```python
from build123d import *

# Parameters (mm, degrees)
CUT_EXTRUDE1_REACH = 53.976
SKETCH2_R          = 3
SKETCH2_R_2        = 2.6


with BuildPart() as part:
    # Sketch1 → Revolve1 (revolve)
    with BuildSketch(Plane.XY, mode=Mode.PRIVATE) as revolve1_sk:
        Polygon((0, -15.5), (29.5, -15.5), (29.5, -9.5), (15, -9.5), (15, 15.5), (0, 15.5), align=None)
    revolve(revolve1_sk.sketch.rotate(Axis((0, 0, 0), (0, -1, 0)), 180), axis=Axis((0, 0, 0), (0, -1, 0)))

    # Sketch2 → Cut-Extrude1 (cut, up to next)
    with BuildSketch(Plane(origin=(0, 15.5, 0), x_dir=(1, 0, 0), z_dir=(0, 1, 0)), mode=Mode.PRIVATE) as cut_extrude1_sk1:
        with Locations(Location((0, 0, 0), (0, 0, 180))):
            Circle(SKETCH2_R)
    cut_extrude1_tool1 = extrude(cut_extrude1_sk1.sketch, amount=-CUT_EXTRUDE1_REACH, mode=Mode.PRIVATE) & part.part
    # Sketch2 → Cut-Extrude1 (cut, up to next)
    with BuildSketch(Plane(origin=(0, 15.5, 0), x_dir=(1, 0, 0), z_dir=(0, 1, 0)), mode=Mode.PRIVATE) as cut_extrude1_sk2:
        with Locations(Location((0, 23.75, 0), (0, 0, 180))):
            Circle(SKETCH2_R_2)
    cut_extrude1_tool2 = extrude(cut_extrude1_sk2.sketch, amount=-CUT_EXTRUDE1_REACH, mode=Mode.PRIVATE) & part.part
    # Sketch2 → Cut-Extrude1 (cut, up to next)
    with BuildSketch(Plane(origin=(0, 15.5, 0), x_dir=(1, 0, 0), z_dir=(0, 1, 0)), mode=Mode.PRIVATE) as cut_extrude1_sk3:
        with Locations(Location((20.56810334, 11.875, 0), (0, 0, 180))):
            Circle(SKETCH2_R_2)
    cut_extrude1_tool3 = extrude(cut_extrude1_sk3.sketch, amount=-CUT_EXTRUDE1_REACH, mode=Mode.PRIVATE) & part.part
    # Sketch2 → Cut-Extrude1 (cut, up to next)
    with BuildSketch(Plane(origin=(0, 15.5, 0), x_dir=(1, 0, 0), z_dir=(0, 1, 0)), mode=Mode.PRIVATE) as cut_extrude1_sk4:
        with Locations(Location((20.56810334, -11.875, 0), (0, 0, 180))):
            Circle(SKETCH2_R_2)
    cut_extrude1_tool4 = extrude(cut_extrude1_sk4.sketch, amount=-CUT_EXTRUDE1_REACH, mode=Mode.PRIVATE) & part.part
    # Sketch2 → Cut-Extrude1 (cut, up to next)
    with BuildSketch(Plane(origin=(0, 15.5, 0), x_dir=(1, 0, 0), z_dir=(0, 1, 0)), mode=Mode.PRIVATE) as cut_extrude1_sk5:
        with Locations(Location((0, -23.75, 0), (0, 0, 180))):
            Circle(SKETCH2_R_2)
    cut_extrude1_tool5 = extrude(cut_extrude1_sk5.sketch, amount=-CUT_EXTRUDE1_REACH, mode=Mode.PRIVATE) & part.part
    # Sketch2 → Cut-Extrude1 (cut, up to next)
    with BuildSketch(Plane(origin=(0, 15.5, 0), x_dir=(1, 0, 0), z_dir=(0, 1, 0)), mode=Mode.PRIVATE) as cut_extrude1_sk6:
        with Locations(Location((-20.56810334, -11.875, 0), (0, 0, 180))):
            Circle(SKETCH2_R_2)
    cut_extrude1_tool6 = extrude(cut_extrude1_sk6.sketch, amount=-CUT_EXTRUDE1_REACH, mode=Mode.PRIVATE) & part.part
    # Sketch2 → Cut-Extrude1 (cut, up to next)
    with BuildSketch(Plane(origin=(0, 15.5, 0), x_dir=(1, 0, 0), z_dir=(0, 1, 0)), mode=Mode.PRIVATE) as cut_extrude1_sk7:
        with Locations(Location((-20.56810334, 11.875, 0), (0, 0, 180))):
            Circle(SKETCH2_R_2)
    cut_extrude1_tool7 = extrude(cut_extrude1_sk7.sketch, amount=-CUT_EXTRUDE1_REACH, mode=Mode.PRIVATE) & part.part
    add(cut_extrude1_tool1.solids().sort_by_distance((0, 15.5, 0))[0], mode=Mode.SUBTRACT)
    add(cut_extrude1_tool2.solids().sort_by_distance((0, 15.5, -23.75))[0], mode=Mode.SUBTRACT)
    add(cut_extrude1_tool3.solids().sort_by_distance((20.568103, 15.5, -11.875))[0], mode=Mode.SUBTRACT)
    add(cut_extrude1_tool4.solids().sort_by_distance((20.568103, 15.5, 11.875))[0], mode=Mode.SUBTRACT)
    add(cut_extrude1_tool5.solids().sort_by_distance((0, 15.5, 23.75))[0], mode=Mode.SUBTRACT)
    add(cut_extrude1_tool6.solids().sort_by_distance((-20.568103, 15.5, 11.875))[0], mode=Mode.SUBTRACT)
    add(cut_extrude1_tool7.solids().sort_by_distance((-20.568103, 15.5, -11.875))[0], mode=Mode.SUBTRACT)


solid = part.part
```
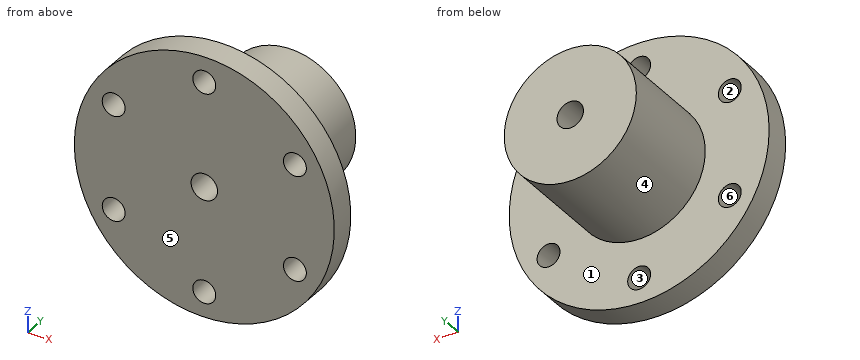
Could you check a few things on this model? Use its own coordinates, in mm. Face numbers are marked on the shaded views. A direction names the side the tool comes from. Round coordinates to 2 decimals unless told otherwise and drop trailing zeros. Order: outer loops, then holes, each group sorted by start corner. A loop starts at its lowest first (then second) coordinate and runs counter-clockwise, first axis right, second up. Notation, with made-up numbers: M 30,-12.75 L 68,-12.75 A11 ccw 68,1.25 Z; hole C 0.5,37.5 d11. An arc over 180 degrees is marked long. One line per question, with ' | ' between items. Start each with the question number.
(1) Suppose I cut it at B-B on z = 0. List the corners of the cut face in (x, y) for me.
(2) Please list where these lines run through material, in increasing order: line 1 along Z through (x, y) = (0, -12); line 2 along Z through (x, y) = (0, 9); line 3 along X through (y, z) = (-11, -10).
(3) Suppose I cut it at C-C on x = -19. List the corners of the cut face in (y, z) for me.
(4) For the marked faces 1 and 2, which set-ups out of +Z, -Z, +X, -X, +Y, -Y let a thin tool reach every point of the face, with its end or its side?
(5) Thinking about a two-plate mould opening in Z: for the marked faces 3, 4, 5 and 6, which applies, +Z half, -Z half, draft (parallel to the pull), parting line (faces both ways), or undercut?
(6) Suppose I cut it at A-A on x = 0. List the corners of the cut face in (y, z) for me, then the cut area to 3 significant figures.
(7) For P1, Ø10, axis at x = -16, y = 2.5, coming from the +Z side; P2, Ø6, axis at x = -20.57, z = -11.88, coming from the +Y side; P3, Ø12, axis at y = 6, z = -7.5, coming from the -X side; P4, Ø7, axis at x = 0, z = 0, coming from the +Y side, each with a flat end and sliding along its axis, tell me the tip position at first contact or that it passes through.
(8) Suppose I cut it at D-D on y = -2. List the corners of the cut face in (x, z) for me.
Geometry results:
1) outline: M -29.5,-15.5 L -3,-15.5 L -3,15.5 L -15,15.5 L -15,-9.5 L -29.5,-9.5 Z; M 3,-15.5 L 29.5,-15.5 L 29.5,-9.5 L 15,-9.5 L 15,15.5 L 3,15.5 Z
2) line 1: -29.5 to -26.35, -21.15 to -3, 3 to 21.15, 26.35 to 29.5 | line 2: -15 to -3, 3 to 15 | line 3: -27.75 to -22.37, -18.77 to 18.77, 22.37 to 27.75
3) outline: M -15.5,-22.57 L -9.5,-22.57 L -9.5,-13.95 L -15.5,-13.95 Z; M -15.5,-9.8 L -9.5,-9.8 L -9.5,9.8 L -15.5,9.8 Z; M -15.5,13.95 L -9.5,13.95 L -9.5,22.57 L -15.5,22.57 Z
4) face 1: +Y | face 2: +Y, -Y
5) face 3: undercut | face 4: parting line | face 5: draft | face 6: undercut
6) outline: M -15.5,-29.5 L -9.5,-29.5 L -9.5,-26.35 L -15.5,-26.35 Z; M -15.5,-21.15 L -9.5,-21.15 L -9.5,-15 L 15.5,-15 L 15.5,-3 L -15.5,-3 Z; M -15.5,3 L 15.5,3 L 15.5,15 L -9.5,15 L -9.5,21.15 L -15.5,21.15 Z; M -15.5,26.35 L -9.5,26.35 L -9.5,29.5 L -15.5,29.5 Z | area: 856 mm²
7) P1: z = 10.2 | P2: y = -9.5 | P3: x = -14.92 | P4: y = 15.5
8) outline: C 0,0 d30; hole C 0,0 d6
